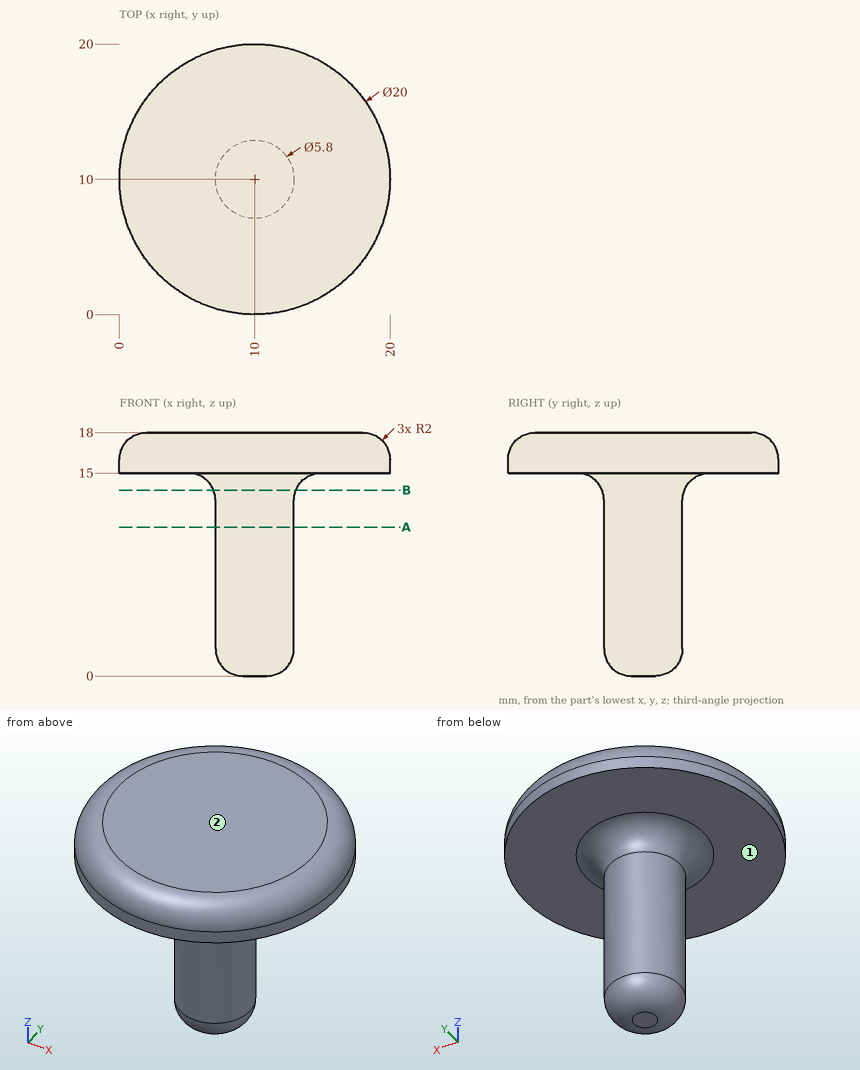
Part print with two shaded views. Sizes in mm from the minimum x, y, z corner. A direction names the side the tool comes from. Give positions to 0.01 mm unless a question says otherwise; leave off trailing zeros. Order: outer loops, then holes, each group sorted by start corner. A loop starts at its lowest first (then second) coordinate and runs counter-clockwise, first axis right, second up.
1) Wall check: probe 1 along Z at (x, y) = (5.5, 16.5); probe 2 along Z at (x, y) = (19, 10.25); probe 3 along Y at (x, z) = (9.5, 10.5). Give the ranges that are in metal, low to high.
2) Pin check, flat tips, straight feed: pin 1 (8 mm diameter, centred on x = 6.5, z = 12.5, fed in from +Y); pin 2 (5 mm diameter, centred on x = 3.5, z = 15.5, fed in from +Y); pin 3 (6 mm diameter, centred on x = 15, z = 10, fed in from -Y). Stop position of each tip, or through.
3) 3-axis set-ups, long thin cutter, end or side, ignore diameter. For the marked faces 1 and 2: which of +Z, -Z, +X, -X, +Y, -Y reach the whole face in a straight line?
4) Saw through at B-B, the plane z = 13.75. Write the cut outline in (x, y), then the cut area to 3 significant figures.
5) Saw through at A-A, the plane z = 11. Write the cut outline in (x, y), then the cut area to 3 significant figures.
Computed:
1. probe 1: z = 15 to 18
1. probe 2: z = 15 to 17.73
1. probe 3: y = 7.14 to 12.86
2. pin 1: stops at y = 19.99
2. pin 2: stops at y = 19.17
2. pin 3: stops at y = 7.9
3. face 1: -Z
3. face 2: +Z, +X, -X, +Y, -Y
4. outline: circle Ø6.09 at (10, 10)
4. area: 29.1 mm2
5. outline: circle Ø5.8 at (10, 10)
5. area: 26.4 mm2
